from build123d import *

# Parameters (mm, degrees)
SKETCH1_R           = 12.5
BOSS_EXTRUDE1_DEPTH = 5
SKETCH2_R           = 3.9
BOSS_EXTRUDE2_DEPTH = 20
SKETCH3_R           = 1.5
CUT_EXTRUDE1_DEPTH  = 3
SKETCH4_R           = 1.25
CUT_EXTRUDE2_DEPTH  = 10


with BuildPart() as part:
    # Sketch1 → Boss-Extrude1 (new body)
    with BuildSketch(Plane.XY):
        Circle(SKETCH1_R)
    extrude(amount=BOSS_EXTRUDE1_DEPTH)

    # Sketch2 → Boss-Extrude2 (add)
    with BuildSketch(Plane(origin=(0, 0, 0), x_dir=(-1, 0, 0), z_dir=(0, 0, -1))):
        Circle(SKETCH2_R)
    extrude(amount=BOSS_EXTRUDE2_DEPTH)

    # Sketch3 → Cut-Extrude1 (cut)
    with BuildSketch(Plane.XY.offset(5)):
        Circle(SKETCH3_R)
    extrude(amount=-CUT_EXTRUDE1_DEPTH, mode=Mode.SUBTRACT)

    # Sketch4 → Cut-Extrude2 (cut)
    with BuildSketch(Plane.XY.offset(5)):
        with Locations((8, 0)):
            Circle(SKETCH4_R)
        with Locations((-8, 0)):
            Circle(SKETCH4_R)
    extrude(amount=-CUT_EXTRUDE2_DEPTH, mode=Mode.SUBTRACT)


solid = part.part
The model under review builds one solid part; all positions refer to its coordinate system, in mm. A direction names the side the tool comes from. Coordinates: 2 decimals unless noted, no trailing zeros. Loops run counter-clockwise (first coordinate to the right, second up) from the corner with the lowest first, then second, coordinate; pieces in that order, holes last. Notation, with made-up numbers: (39.5, 85.5) -> (61.5, 85.5) arc R21 cw to (61.5, 123.5) -> close; hole circle Ø4 at (6.5, 30). An arc over 180 degrees is marked (long way). Use a Markdown table: item, result. Add a question column.
1. Add section C-C on y = -2.5. Write out the cut boundary in (x, z), plus the area to 3 significant figures.
2. Clearance check with flat-ended pins moving along their axes: pin 1 Ø3 at (x, y) = (8, 0) entering from -Z; pin 2 Ø2.5 at (x, y) = (0, 0) entering from +Z; pin 3 Ø5 at (y, z) = (6, -0.5) entering from -X. State where each tip first meets the part, or that it passes through.
3. Draft analysis for pull direction Y (two halves, no side actions). For faces 4 (the face through (0, -3, 5)), 5 (the face through (2.87, 2.64, -9.86)), 6 (the face through (0, 0, 2)), state which applies: pulls with the +Y half, pulls with the -Y half, needs draft (parallel to the pull), parting line crosses it, or undercut.
4. Add section D-D on x = -8. Write out the cut boundary in (y, z).
5. Machinability: for faces 1 (the face through (0, 0, -20)), 2 (the face through (3, 3, 0)), 3 (the face through (-1.5, 0.07, 3.52)), which of the approach directions +Z, -Z, +X, -X, +Y, -Y give a long, thin tool a straight path to every point of the face, cutting with its end or side? Answer none if there is none.
6. Add section A-A on y = 0. Write out the cut boundary in (x, z).
7. Add section B-B on x = 0. Write out the cut boundary in (y, z).
8. To check wall thickness, follow line 1 (Y direction, x = 0, z = 3.35); line 2 (Z direction, x = 9.5, y = -0.25); line 3 (X direction, y = -0.25, z = -10). State the ranges of each line that lie inside material, in increasing order.
Returned:
| question | item | result |
|---|---|---|
| 1 | outline | (-12.25, 0) -> (-2.99, 0) -> (-2.99, -20) -> (2.99, -20) -> (2.99, 0) -> (12.25, 0) -> (12.25, 5) -> (-12.25, 5) -> close |
| 1 | area | 242 mm² |
| 2 | pin 1 | stops at z = 0 |
| 2 | pin 2 | stops at z = 2 |
| 2 | pin 3 | stops at x = -11.99 |
| 3 | face 4 | needs draft |
| 3 | face 5 | parting line crosses it |
| 3 | face 6 | undercut |
| 4 | outline | (-9.6, 0) -> (-1.25, 0) -> (-1.25, 5) -> (-9.6, 5) -> close; (1.25, 0) -> (9.6, 0) -> (9.6, 5) -> (1.25, 5) -> close |
| 5 | face 1 | -Z, +X, -X, +Y, -Y |
| 5 | face 2 | -Z |
| 5 | face 3 | +Z |
| 6 | outline | (-12.5, 0) -> (-9.25, 0) -> (-9.25, 5) -> (-12.5, 5) -> close; (-6.75, 0) -> (-3.9, 0) -> (-3.9, -20) -> (3.9, -20) -> (3.9, 0) -> (6.75, 0) -> (6.75, 5) -> (1.5, 5) -> (1.5, 2) -> (-1.5, 2) -> (-1.5, 5) -> (-6.75, 5) -> close; (9.25, 0) -> (12.5, 0) -> (12.5, 5) -> (9.25, 5) -> close |
| 7 | outline | (-12.5, 0) -> (-3.9, 0) -> (-3.9, -20) -> (3.9, -20) -> (3.9, 0) -> (12.5, 0) -> (12.5, 5) -> (1.5, 5) -> (1.5, 2) -> (-1.5, 2) -> (-1.5, 5) -> (-12.5, 5) -> close |
| 8 | line 1 | y = -12.5 to -1.5, 1.5 to 12.5 |
| 8 | line 2 | z = 0 to 5 |
| 8 | line 3 | x = -3.89 to 3.89 |
